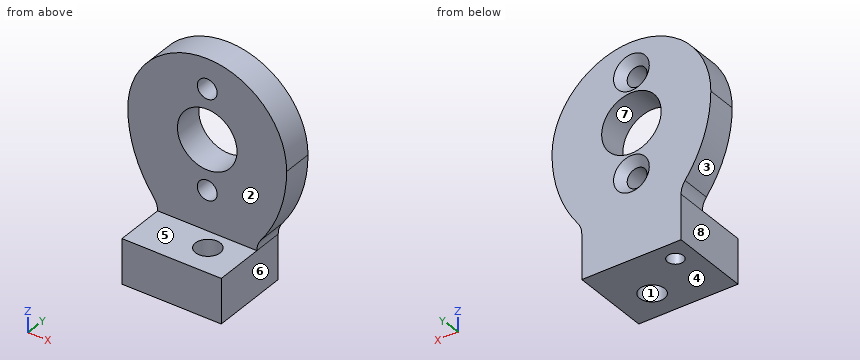
```python
from build123d import *

# Parameters (mm, degrees)
BOSS_EXTRUDE1_DEPTH           = 3
SKETCH2_W                     = 10
SKETCH2_H                     = 4.5
BOSS_EXTRUDE2_DEPTH           = 5
F_6_0_6_DIAMETER_HOLE1_D      = 6
M3X0_5_TAPPED_HOLE1_D         = 2.5
M2X0_4_TAPPED_HOLE1_D         = 1.6
M2X0_4_TAPPED_HOLE1_DEPTH     = 5.2
M2X0_4_TAPPED_HOLE1_TIP       = 0.480688495
FILLET1_R                     = 2
CSK_FOR_M3_SFHCS3_D           = 2
CSK_FOR_M3_SFHCS3_DEPTH       = 9.5
CSK_FOR_M3_SFHCS3_CSINK_D     = 3.6
CSK_FOR_M3_SFHCS3_CSINK_ANGLE = 90
CSK_FOR_M3_SFHCS3_TIP         = 0.600860619


with BuildPart() as part:
    # Sketch1 → Boss-Extrude1 (new body)
    with BuildSketch(Plane(origin=(0, 3, 0), x_dir=(1, 0, 0), z_dir=(0, 1, 0))):
        with BuildLine():
            Line((5.000000003, -5.193376137), (5.000000003, 0))
            Line((5.000000003, 0), (-4.999999997, 0))
            Line((-4.999999997, 0), (-4.999999997, -5.193376137))
            ThreePointArc((-4.999999997, -5.193376137), (-7.227019257, -9.084119567), (-7.999999997, -13.5))
            ThreePointArc((-7.999999997, -13.5), (3e-09, -21.5), (8.000000003, -13.5))
            ThreePointArc((8.000000003, -13.5), (7.227019264, -9.084119567), (5.000000003, -5.193376137))
        make_face()
    extrude(amount=-BOSS_EXTRUDE1_DEPTH)

    # Sketch2 → Boss-Extrude2 (add)
    with BuildSketch(Plane.XZ):
        with Locations((0, 2.25)):
            Rectangle(SKETCH2_W, SKETCH2_H)
    extrude(amount=BOSS_EXTRUDE2_DEPTH)

    # Ø6.0 (6) Diameter Hole1 (through all)
    with Locations(Plane(origin=(0, 0, 0), x_dir=(-1, 0, 0), z_dir=(0, -1, 0))):
        with Locations((0, -13.5)):
            Hole(F_6_0_6_DIAMETER_HOLE1_D / 2)

    # M3x0.5 Tapped Hole1 (through all)
    with Locations(Plane(origin=(0, 0, 0), x_dir=(-1, 0, 0), z_dir=(0, 0, -1))):
        with Locations((-1.5, -2)):
            Hole(M3X0_5_TAPPED_HOLE1_D / 2)

    # M2x0.4 Tapped Hole1
    with Locations(Plane(origin=(0, 0, 0), x_dir=(-1, 0, 0), z_dir=(0, 0, -1))):
        with Locations((3, 1)):
            Hole(M2X0_4_TAPPED_HOLE1_D / 2, depth=M2X0_4_TAPPED_HOLE1_DEPTH)
            with Locations((0, 0, -(M2X0_4_TAPPED_HOLE1_DEPTH + M2X0_4_TAPPED_HOLE1_TIP / 2))):  # 118° drill point
                Cone(0, M2X0_4_TAPPED_HOLE1_D / 2, M2X0_4_TAPPED_HOLE1_TIP, mode=Mode.SUBTRACT)

    # Fillet1
    fillet1_edges = [part.edges().sort_by_distance(p)[0] for p in [
        (5.000000003, 1.5, 5.193376137),
        (-4.999999997, 1.5, 5.193376137),
    ]]
    fillet(fillet1_edges, radius=FILLET1_R)

    # CSK for M3 SFHCS3
    with Locations(Plane(origin=(3e-09, 3, 8.5), x_dir=(0, 0, 1), z_dir=(0, 1, 0))):
        with Locations((0, 0), (10, 0)):
            CounterSinkHole(CSK_FOR_M3_SFHCS3_D / 2, CSK_FOR_M3_SFHCS3_CSINK_D / 2, depth=CSK_FOR_M3_SFHCS3_DEPTH, counter_sink_angle=CSK_FOR_M3_SFHCS3_CSINK_ANGLE)
            with Locations((0, 0, -(CSK_FOR_M3_SFHCS3_DEPTH + CSK_FOR_M3_SFHCS3_TIP / 2))):  # 118° drill point
                Cone(0, CSK_FOR_M3_SFHCS3_D / 2, CSK_FOR_M3_SFHCS3_TIP, mode=Mode.SUBTRACT)


solid = part.part
```
Design review of the part built by this model. Coordinates are the model's own, in mm. Face numbers are marked on the shaded views. A direction names the side the tool comes from. Coordinates: 2 decimals unless noted, no trailing zeros. Loops run counter-clockwise (first coordinate to the right, second up) from the corner with the lowest first, then second, coordinate; pieces in that order, holes last. Notation, with made-up numbers: (77, 48.5) - (109, 48.5) arc R8 cw to (109, 54.5) - close; hole circle Ø10 at (26, -35.75). An arc over 180 degrees is marked (long way). Use CSV: the item, a comma, the result in double quotes. Start each with the question number.
1) Consider section D-D on y = -1. Write out the cut boundary in (x, z), then the cut area to 4 significant figures.
2) Wall thickness on L1, parallel to Y at x = -3, z = 2.2; L2, parallel to Y at x = -6, z = 17.75; L3, parallel to Y at x = 1.5, z = 2.4: over which ranges is each line inside the solid? List them lowest first. Write a range as from..to.
3) Tool access review of the marked faces 4, 5, 6, 7 and 8: name each direction out of +Z, -Z, +X, -X, +Y, -Y from which nothing blocks a thin tool from reaching the whole face with its end or side.
4) Consider section B-B on z = 8.5. Write out the cut boundary in (x, y).
5) The part is to be moulded in two halves that separate along X. For the marked faces 1, 2 and 3, say which applies: +X half, -X half, draft (parallel to the pull), parting line (faces both ways), or undercut.
6) For pin 1 Ø3 at (y, z) = (2, 2.5) entering from +X; pin 2 Ø1.6 at (x, z) = (0, 8.5) entering from -Y; pin 3 Ø2.5 at (x, z) = (0, 18.5) entering from -Y; pin 4 Ø3 at (y, z) = (-1, 11.5) entering from +X, all flat-tipped, find the tip position at first contact; note any pin that passes through.
7) Consider section A-A on y = -2.75. Write out the cut boundary in (x, z), then the cut area to 3 significant figures.
8) Consider section C-C on x = 0. Write out the cut boundary in (y, z), then the cut area to 3 significant figures.
Geometry says:
1,outline,"(-5, 0) - (0.75, 0) - (0.75, 4.5) - (-5, 4.5) - close; (2.25, 0) - (5, 0) - (5, 4.5) - (2.25, 4.5) - close"
1,area,"38.25 mm^2"
2,L1,"-5..0.2, 1.8..3"
2,L2,"0..3"
2,L3,"-5..-3.25, -0.75..3"
3,face 4,"-Z, +X, -X, +Y, -Y"
3,face 5,"+Z, +X, -X, -Y"
3,face 6,"-Z, +X, +Y, -Y"
3,face 7,"+Y, -Y"
3,face 8,"-Z, -X, +Y, -Y"
4,outline,"(-7, 0) - (-1, 0) - (-1, 2.2) - (-1.8, 3) - (-7, 3) - close; (1, 0) - (7, 0) - (7, 3) - (1.8, 3) - (1, 2.2) - close"
5,face 1,"undercut"
5,face 2,"draft"
5,face 3,"-X half"
6,pin 1,"x = 5"
6,pin 2,"through"
6,pin 3,"y = 0"
6,pin 4,"x = 7.97"
7,outline,"(-5, 0) - (0.5, 0) - (0.5, 4.5) - (-5, 4.5) - close; (2.5, 0) - (5, 0) - (5, 4.5) - (2.5, 4.5) - close"
7,area,"36.0 mm^2"
8,outline,"(-5, 0) - (3, 0) - (3, 6.7) - (2.2, 7.5) - (0, 7.5) - (0, 4.5) - (-5, 4.5) - close; (0, 9.5) - (2.2, 9.5) - (3, 10.3) - (3, 10.5) - (0, 10.5) - close; (0, 16.5) - (3, 16.5) - (3, 16.7) - (2.2, 17.5) - (0, 17.5) - close; (0, 19.5) - (2.2, 19.5) - (3, 20.3) - (3, 21.5) - (0, 21.5) - close"
8,area,"55.7 mm^2"
